Geometry: final body of the model. Coordinates: model frame, mm. Face numbers are marked on the shaded views. A direction names the side the tool comes from. Round coordinates to 2 decimals unless told otherwise and drop trailing zeros. Write each loop counter-clockwise with the first axis right and the second up, starting at its lowest first coordinate (ties: lowest second). Pieces come first, ordered by that corner, then holes. Notation, with made-up numbers: M -15,26 L 39,26 A25 ccw 39,61 Z; hole C -29,2.25 d7. An arc over 180 degrees is marked long. Answer as CSV lines item,"result". Start each with the question number.
Q1. Ray query, probe 1 along Y at (x, z) = (17.5, 25); probe 2 along Y at (x, z) = (6.5, 10); probe 3 along X at (y, z) = (28, -17.5). Return the intervals inside material, ascending.
Q2. Reachability of the marked faces 1 and 2 from +Z, -Z, +X, -X, +Y, -Y: full face, straight path, thin tool, end or side. Return the list, or none.
Q3. Section query A-A on x = 0. Output: boundary loops of the cut face in (y, z).
Q4. Section query B-B on y = 19. Output: boundary loops of the cut face in (x, z), and give its area (3 significant figures).
Q5. First-contact query: pin 1 (1.5 mm diameter, centred on x = 14, y = -4.5, fed in from +Z); pin 2 (2 mm diameter, centred on x = -24.5, z = 24, fed in from -Y); pin 3 (10 mm diameter, centred on x = -8, z = 14, fed in from -Y). Flat tips, straight axial feed; report the tip coordinate or a pass-through.
```python
from build123d import *

# Parameters (mm, degrees)
SKETCH1_R           = 26
BOSS_EXTRUDE1_DEPTH = 29
SKETCH2_W           = 60
SKETCH2_H           = 60
BOSS_EXTRUDE2_DEPTH = 11.6
FILLET1_R           = 5
SKETCH5_R           = 2
BOSS_EXTRUDE3_DEPTH = 10
SKETCH6_R           = 1
BOSS_EXTRUDE4_DEPTH = 9
FILLET2_R           = 1
FILLET3_R           = 1
SKETCH7_R           = 5
BOSS_EXTRUDE5_DEPTH = 1


with BuildPart() as part:
    # Sketch1 → Boss-Extrude1 (new body)
    with BuildSketch(Plane(origin=(0, 0, 0), x_dir=(1, 0, 0), z_dir=(0, 1, 0))):
        with Locations(Location((0, 0, 0), (0, 0, 90))):
            Circle(SKETCH1_R)
    extrude(amount=BOSS_EXTRUDE1_DEPTH)

    # Sketch2 → Boss-Extrude2 (add)
    with BuildSketch(Plane(origin=(0, 29, 0), x_dir=(1, 0, 0), z_dir=(0, 1, 0))):
        Rectangle(SKETCH2_W, SKETCH2_H)
    extrude(amount=BOSS_EXTRUDE2_DEPTH)

    # Fillet1
    fillet1_edges = [part.edges().sort_by_distance(p)[0] for p in [
        (30, 34.8, 30),
        (30, 34.8, -30),
        (-30, 34.8, -30),
        (-30, 34.8, 30),
    ]]
    fillet(fillet1_edges, radius=FILLET1_R)

    # Sketch5 → Boss-Extrude3 (add)
    with BuildSketch(Plane.XZ):
        with Locations(Location((15, -10, 0), (0, 0, 90))):
            Circle(SKETCH5_R)
        with Locations(Location((-15, -10, 0), (0, 0, 90))):
            Circle(SKETCH5_R)
    extrude(amount=BOSS_EXTRUDE3_DEPTH)

    # Sketch6 → Boss-Extrude4 (add)
    with BuildSketch(Plane.XZ.offset(-29)):
        with Locations(Location((24, -24, 0), (0, 0, 270))):
            Circle(SKETCH6_R)
        with Locations(Location((24, 24, 0), (0, 0, 90))):
            Circle(SKETCH6_R)
        with Locations(Location((-24, 24, 0), (0, 0, 270))):
            Circle(SKETCH6_R)
        with Locations(Location((-24, -24, 0), (0, 0, 90))):
            Circle(SKETCH6_R)
    extrude(amount=BOSS_EXTRUDE4_DEPTH)

    # Fillet2
    fillet2_edges = [part.edges().sort_by_distance(p)[0] for p in [
        (-30, 40.6, 0),
        (0, 40.6, -30),
        (30, 40.6, 0),
        (0, 40.6, 30),
        (28.535533906, 40.6, 28.535533906),
        (28.535533906, 40.6, -28.535533906),
        (-28.535533906, 40.6, 28.535533906),
        (-28.535533906, 40.6, -28.535533906),
    ]]
    fillet(fillet2_edges, radius=FILLET2_R)

    # Fillet3
    fillet3_edges = [part.edges().sort_by_distance(p)[0] for p in [
        (0, 0, 26),
    ]]
    fillet(fillet3_edges, radius=FILLET3_R)

    # Sketch7 → Boss-Extrude5 (add)
    with BuildSketch(Plane.XZ):
        with Locations(Location((15, -10, 0), (0, 0, 90))):
            Circle(SKETCH7_R)
        with Locations(Location((-15, -10, 0), (0, 0, 90))):
            Circle(SKETCH7_R)
    extrude(amount=BOSS_EXTRUDE5_DEPTH)


solid = part.part
```
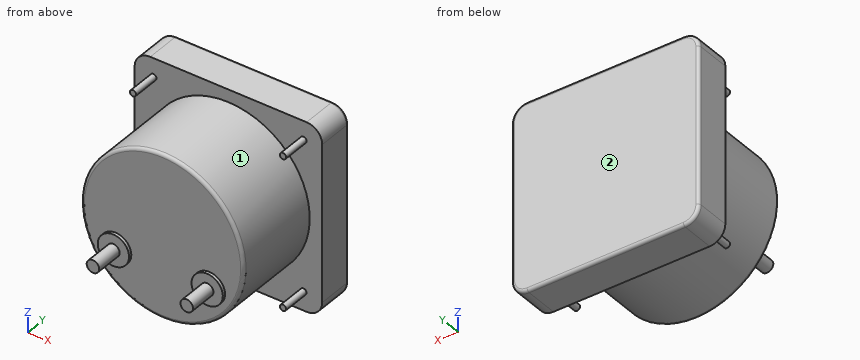
Entries:
1,probe 1,"y = 29 to 40.6"
1,probe 2,"y = 0 to 40.6"
1,probe 3,"x = -19.23 to 19.23"
2,face 1,"-Y"
2,face 2,"+Z, -Z, +X, -X, +Y"
3,outline,"M 0,-25 A1 ccw 1,-26 L 29,-26 L 29,-30 L 39.6,-30 A1 ccw 40.6,-29 L 40.6,29 A1 ccw 39.6,30 L 29,30 L 29,26 L 1,26 A1 ccw 0,25 Z"
4,outline,"C 0,0 d52"
4,area,"2,120 mm^2"
5,pin 1,"stops at z = -8.02"
5,pin 2,"stops at y = 20"
5,pin 3,"stops at y = 0"
